from build123d import *

# Parameters (mm, degrees)
SKETCH_1_R          = 12.5
EXTRUDE_1_DEPTH     = 10
SKETCH_2_R          = 20
SKETCH_2_R_2        = 12.5
EXTRUDE_2_DEPTH     = 43
SKETCH_3_R          = 3.3
CUT_EXTRUDE_1_DEPTH = 59.457249337
SKETCH_4_R          = 3
CUT_EXTRUDE_2_DEPTH = 59.457249337


with BuildPart() as part:
    # 草图1 → 凸台-拉伸1 (new body)
    with BuildSketch(Plane(origin=(0, 0, 0), x_dir=(1, 0, 0), z_dir=(0, 1, 0))):
        with BuildLine():
            Line((-24, 20.402205763), (-24, -20.402205763))
            ThreePointArc((-24, -20.402205763), (0, -31.5), (24, -20.402205763))
            Line((24, -20.402205763), (24, 20.402205763))
            ThreePointArc((24, 20.402205763), (0, 31.5), (-24, 20.402205763))
        make_face()
        with Locations(Location((0, 0, 0), (0, 0, 270))):
            Circle(SKETCH_1_R, mode=Mode.SUBTRACT)
    extrude(amount=-EXTRUDE_1_DEPTH)

    # 草图2 → 凸台-拉伸2 (add)
    with BuildSketch(Plane(origin=(0, 0, 0), x_dir=(1, 0, 0), z_dir=(0, 1, 0))):
        with Locations(Location((0, 0, 0), (0, 0, 270))):
            Circle(SKETCH_2_R)
        with Locations(Location((0, 0, 0), (0, 0, 270))):
            Circle(SKETCH_2_R_2, mode=Mode.SUBTRACT)
    extrude(amount=-EXTRUDE_2_DEPTH)

    # 草图3 → 切除-拉伸1 (cut, through all)
    with BuildSketch(Plane(origin=(0, 0, 0), x_dir=(1, 0, 0), z_dir=(0, 1, 0))):
        with Locations(Location((0, 25.5, 0), (0, 0, 270))):
            Circle(SKETCH_3_R)
        with Locations(Location((-18.03122292, 18.03122292, 0), (0, 0, 270))):
            Circle(SKETCH_3_R)
        with Locations(Location((18.03122292, 18.03122292, 0), (0, 0, 270))):
            Circle(SKETCH_3_R)
        with Locations(Location((18.03122292, -18.03122292, 0), (0, 0, 270))):
            Circle(SKETCH_3_R)
        with Locations(Location((-18.03122292, -18.03122292, 0), (0, 0, 270))):
            Circle(SKETCH_3_R)
        with Locations(Location((0, -25.5, 0), (0, 0, 270))):
            Circle(SKETCH_3_R)
    extrude(amount=-CUT_EXTRUDE_1_DEPTH, mode=Mode.SUBTRACT)

    # 草图4 → 切除-拉伸2 (cut, through all)
    with BuildSketch(Plane(origin=(0, 0, 0), x_dir=(0, 0, -1), z_dir=(1, 0, 0))):
        with Locations((0, -5)):
            Circle(SKETCH_4_R)
    extrude(amount=-CUT_EXTRUDE_2_DEPTH, mode=Mode.SUBTRACT)


solid = part.part
Source: CAD feature listing. Evaluate the final solid. Frame: model axes, mm. A direction names the side the tool comes from. Give positions to 0.01 mm unless a question says otherwise; leave off trailing zeros. Write each loop counter-clockwise with the first axis right and the second up, starting at its lowest first coordinate (ties: lowest second). Pieces come first, ordered by that corner, then holes. Notation, with made-up numbers: (51.5, 88.5) -> (108.5, 88.5) arc R38 cw to (108.5, 126.5) -> close; hole circle Ø8 at (-15, 3). An arc over 180 degrees is marked (long way). Return JSON: item names as keys, results as strings. Group by question number.
1. Section A-A, the plane z = 0. Output: boundary loops of the cut face in (x, y), then the cut area to 3 significant figures.
2. Access query for faces 5 (the face through (-17.04, -4.93, -14.884)), 6 (the face through (-18, -2, 0)). Directions: +Z, -Z, +X, -X, +Y, -Y. A direction counts if a zero-diameter tool reaches every point of the face in a straight line with its end or side. Return the directions, or none.
3. Section B-B, the plane x = 0. Output: boundary loops of the cut face in (y, z), then the cut area to 3 significant figures.
4. Mould query, pull axis Z, two halves, no side actions, for faces 1 (the face through (-1.26, -4.93, 28.55)), 2 (the face through (0, -10, -21)), 3 (the face through (-19.524, -26.269, -4.336)), 4 (the face through (20.814, -4.93, -16.257)). Classes: +Z half, -Z half, draft (parallel to the pull), parting line (faces both ways), or undercut.
5. Pin query (flat end, axial travel): pin 1 Ø8 at (x, y) = (4, -21) entering from -Z; pin 2 Ø10 at (x, y) = (16, -10.5) entering from -Z; pin 3 Ø2 at (x, y) = (4, -17) entering from -Z. Return the tip coordinate at first contact, or that it passes through.
6. Section D-D, the plane z = 25.5. Output: boundary loops of the cut face in (x, y), then the cut area to 3 significant figures.
7. Material intervals for line 1 (Z direction, x = -15, y = -8.5); line 2 (X direction, y = -28.5, z = 0.5); line 3 (Y direction, x = -18.5, z = 0), sorted ascending. Write a range as from..to.
8. Section C-C, the plane y = -5. Output: boundary loops of the cut face in (x, z), then the cut area to 3 significant figures.
Determined:
{
 "1": {"outline": "(-24, -10) -> (-20, -10) -> (-20, -43) -> (-12.5, -43) -> (-12.5, -8) -> (-24, -8) -> close; (-24, -2) -> (-12.5, -2) -> (-12.5, 0) -> (-24, 0) -> close; (12.5, -43) -> (20, -43) -> (20, -10) -> (24, -10) -> (24, 0) -> (12.5, 0) -> close", "area": "656 mm2"},
 "2": {"face 5": "+Y, -Y", "face 6": "-X"},
 "3": {"outline": "(-43, -20) -> (-10, -20) -> (-10, -22.2) -> (0, -22.2) -> (0, -12.5) -> (-43, -12.5) -> close; (-43, 12.5) -> (0, 12.5) -> (0, 22.2) -> (-10, 22.2) -> (-10, 20) -> (-43, 20) -> close; (-10, -31.5) -> (0, -31.5) -> (0, -28.8) -> (-10, -28.8) -> close; (-10, 28.8) -> (0, 28.8) -> (0, 31.5) -> (-10, 31.5) -> close", "area": "743 mm2"},
 "4": {"face 1": "undercut", "face 2": "draft", "face 3": "parting line", "face 4": "undercut"},
 "5": {"pin 1": "stops at z = -20", "pin 2": "stops at z = -29.51", "pin 3": "stops at z = -19.77"},
 "6": {"outline": "(-18.49, -10) -> (-3.3, -10) -> (-3.3, 0) -> (-18.49, 0) -> close; (3.3, -10) -> (18.49, -10) -> (18.49, 0) -> (3.3, 0) -> close", "area": "304 mm2"},
 "7": {"line 1": "z = -27.7..-19.34, -16.73..16.73, 19.34..27.7", "line 2": "x = -19.99..-12.49, 12.49..19.99", "line 3": "y = -43..-8, -2..0"},
 "8": {"outline": "(-24, -20.4) arc R31.5 ccw to (24, -20.4) -> (24, 20.4) arc R31.5 ccw to (-24, 20.4) -> (-24, 3) -> (-12.13, 3) arc R12.5 cw (long way) to (-12.13, -3) -> (-24, -3) -> close; hole circle Ø6.6 at (-18.03, -18.03); hole circle Ø6.6 at (-18.03, 18.03); hole circle Ø6.6 at (0, -25.5); hole circle Ø6.6 at (0, 25.5); hole circle Ø6.6 at (18.03, -18.03); hole circle Ø6.6 at (18.03, 18.03)", "area": "1,930 mm2"}
}
